Can you work these out from the model? Positions are in its coordinate system, mm. A direction names the side the tool comes from. Give positions to 0.01 mm unless a question says otherwise; leave off trailing zeros. Loops run counter-clockwise (first coordinate to the right, second up) from the corner with the lowest first, then second, coordinate; pieces in that order, holes last. Notation, with made-up numbers: (-37, 50) -> (-18, 50) arc R9 ccw to (-18, 66) -> close; hole circle Ø9 at (33.5, -40). An arc over 180 degrees is marked (long way). Return JSON: item names as keys, results as strings. Group by question number.
Q1. Will these pins go through, and if not, where does the flat tip stop? pin 1 (1.4 mm diameter, centred on y = 7, z = 3, fed in from +X); pin 2 (1.4 mm diameter, centred on y = -7, z = 3, fed in from -X); pin 3 (5 mm diameter, centred on y = 5, z = 2.5, fed in from -X); pin 4 (18 mm diameter, centred on x = 0, y = 0, fed in from -Z).
Q2. I need wall thicknesses on line 1 along X through (y, z) = (0, 0.25) (3 decimals); line 2 along Y through (x, z) = (26, 1.75). Which ranges of each line are inside material? Lowest first, please. Write a range as [from, to].
Q3. Suppose I cut it at C-C, the plane y = 31. Please give me the cut outline in (x, z), and give its area (3 significant figures).
Q4. Which directions (+Z, -Z, +X, -X, +Y, -Y) give clear straight access to the entire face, cutting with the end or side of a thin tool? Please do faces 1 (the flat face through (-23.9, -31, 0)), 2 (the flat face through (-31.2, 6.9, 0)), 3 (the flat face through (23.9, 31, 0)).
Q5. Suppose I cut it at D-D, the plane x = -20.5. Please give me the cut outline in (y, z).
Q6. Suppose I cut it at A-A, the plane y = 0. Please give me the cut outline in (x, z) (3 decimals).
Q7. Thinking about a two-plate mould opening in X: for faces 4 (the cylindrical face through (-36.174, -36.142, 0.036)), 5 (the cylindrical face through (-36.142, 36.174, 0.036)), 6 (the flat face through (-12, 4, -5.08)), 7 (the flat face through (31, -23.9, 0)), which applies, pulls with the +X half, pulls with the -X half, needs draft (parallel to the pull), parting line crosses it, or undercut?
```python
from build123d import *

# Parameters (mm, degrees)
F1_DEPTH = 5.08
F2_R     = 1.27
F3_DEPTH = 2.54
F4_R     = 1.27


with BuildPart() as f1:
    # F0 (on Top) → F1 (new body, symmetric)
    with BuildSketch(Plane.XY):
        with BuildLine():
            Line((19.05, 19.05), (-19.05, 19.05))
            Line((-19.05, 19.05), (-19.05, 0))
            Line((-19.05, 0), (-11.125, 0))
            ThreePointArc((-11.125, 0), (0, 11.125), (11.125, 0))
            Line((11.125, 0), (19.05, 0))
            Line((19.05, 0), (19.05, 19.05))
        make_face()
        with BuildLine():
            Line((-11.125, 0), (-19.05, 0))
            Line((-19.05, 0), (-19.05, -19.05))
            Line((-19.05, -19.05), (19.05, -19.05))
            Line((19.05, -19.05), (19.05, 0))
            Line((19.05, 0), (11.125, 0))
            ThreePointArc((11.125, 0), (0, -11.125), (-11.125, 0))
        make_face()
    extrude(amount=F1_DEPTH, both=True)

    # F2
    f2_edges = [f1.edges().sort_by_distance(p)[0] for p in [
        (19.05, 0, 5.08),
        (0, -19.05, 5.08),
        (-19.05, 0, 5.08),
        (0, 19.05, 5.08),
        (-11.125, 0, 5.08),
        (-11.125, 0, -5.08),
        (19.05, 0, -5.08),
        (0, -19.05, -5.08),
        (0, 19.05, -5.08),
        (-19.05, 0, -5.08),
    ]]
    fillet(f2_edges, radius=F2_R)

    # F0 (on Top) → F3 (join, symmetric)
    with BuildSketch(Plane.XY):
        Polygon((-12.7, -25.4), (-19.05, -19.05), (-25.4, -12.7), (-38.1, -38.1), align=None)
        Polygon((19.05, -19.05), (-19.05, -19.05), (-12.7, -25.4), (0, -38.1), (12.7, -25.4), align=None)
        Polygon((25.4, -12.7), (19.05, -19.05), (12.7, -25.4), (38.1, -38.1), align=None)
        Polygon((38.1, 0), (19.05, 0), (19.05, -19.05), (25.4, -12.7), align=None)
        Polygon((25.4, 12.7), (19.05, 19.05), (19.05, 0), (38.1, 0), align=None)
        Polygon((-12.7, 25.4), (-19.05, 19.05), (19.05, 19.05), (12.7, 25.4), (0, 38.1), align=None)
        Polygon((-19.05, 0), (-19.05, 19.05), (-25.4, 12.7), (-38.1, 0), (-25.4, -12.7), (-19.05, -19.05), align=None)
        Polygon((-25.4, 12.7), (-19.05, 19.05), (-12.7, 25.4), (-38.1, 38.1), align=None)
        Polygon((12.7, 25.4), (19.05, 19.05), (25.4, 12.7), (38.1, 38.1), align=None)
    extrude(amount=F3_DEPTH, both=True)

    # F4
    f4_edges = [f1.edges().sort_by_distance(p)[0] for p in [
        (-38.1, -38.1, 0),
        (-38.1, 0, 0),
        (-38.1, 38.1, 0),
        (0, 38.1, 0),
        (38.1, 38.1, 0),
        (38.1, 0, 0),
        (38.1, -38.1, 0),
        (0, -38.1, 0),
    ]]
    fillet(f4_edges, radius=F4_R)


solid = f1.part
```
Ans:
{
 "1": {"pin 1": "stops at x = 31.63", "pin 2": "stops at x = -31.63", "pin 3": "stops at x = -35.6", "pin 4": "passes through"},
 "2": {"line 1": "x = [-37.574, -11.125], [11.125, 37.574]", "line 2": "y = [-32.05, -13.9], [-12.1, 12.1], [13.9, 32.05]"},
 "3": {"outline": "(-34.55, -2.54) -> (-23.9, -2.54) -> (-23.9, 2.54) -> (-34.55, 2.54) -> close; (-7.1, -2.54) -> (7.1, -2.54) -> (7.1, 2.54) -> (-7.1, 2.54) -> close; (23.9, -2.54) -> (34.55, -2.54) -> (34.55, 2.54) -> (23.9, 2.54) -> close", "area": "180 mm^2"},
 "4": {"face 1": "+Z, -Z, -Y", "face 2": "+Z, -Z, -X", "face 3": "+Z, -Z, +Y"},
 "5": {"outline": "(-29.3, -2.54) -> (29.3, -2.54) -> (29.3, 2.54) -> (-29.3, 2.54) -> close"},
 "6": {"outline": "(-37.574, -2.54) -> (-19.05, -2.54) -> (-19.05, -3.81) arc R1.27 ccw to (-17.78, -5.08) -> (-12.395, -5.08) arc R1.27 ccw to (-11.125, -3.81) -> (-11.125, 3.81) arc R1.27 ccw to (-12.395, 5.08) -> (-17.78, 5.08) arc R1.27 ccw to (-19.05, 3.81) -> (-19.05, 2.54) -> (-37.574, 2.54) -> close; (11.125, -3.81) arc R1.27 ccw to (12.395, -5.08) -> (17.78, -5.08) arc R1.27 ccw to (19.05, -3.81) -> (19.05, -2.54) -> (37.574, -2.54) -> (37.574, 2.54) -> (19.05, 2.54) -> (19.05, 3.81) arc R1.27 ccw to (17.78, 5.08) -> (12.395, 5.08) arc R1.27 ccw to (11.125, 3.81) -> close"},
 "7": {"face 4": "undercut", "face 5": "undercut", "face 6": "needs draft", "face 7": "pulls with the +X half"}
}
